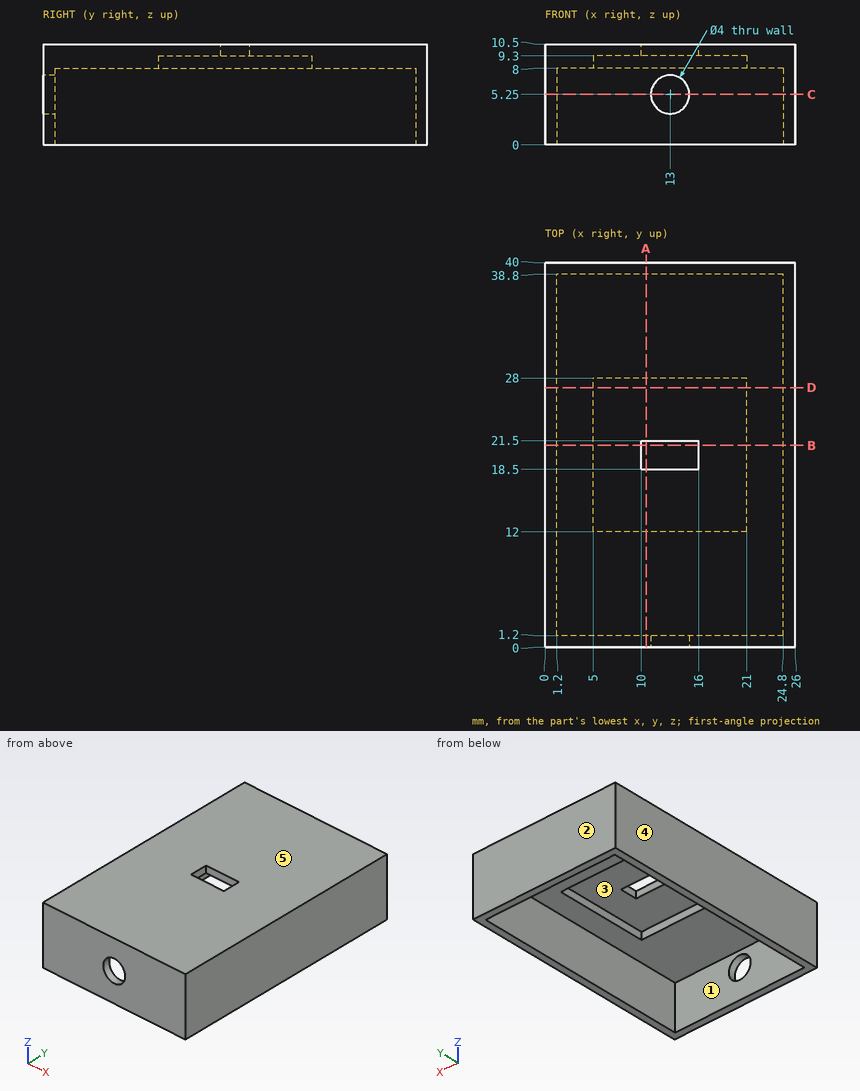
Study the drawing (mm; zero at the part's minimum x, y, z) and answer. A direction names the side the tool comes from. Round coordinates to 2 decimals unless told otherwise and drop trailing zeros. Order: outer loops, then holes, each group sorted by start corner. A loop starts at its lowest first (then second) coordinate and runs counter-clockwise, first axis right, second up. Notation, with made-up numbers: M -2,50.25 L 2,50.25 A32 cw 2,86.25 Z; hole C -7,59 d6. An arc over 180 degrees is marked long. One line per item, written item: value.
Q1. Flat-ended cylindrical pins translate along their axes: pin 1 (5 mm diameter, centred on x = 20, y = 17, fed in from -Z); pin 2 (5 mm diameter, centred on x = 16, y = 23.5, fed in from -Z). Find the tip coordinate at first contact, or state that the pin passes through.
Derived:
pin 1: z = 8
pin 2: z = 9.3
Q2. Determine the mould class of the marked faces 3, 4 and 5 for opening direction X: released by +X, released by -X, zero draft, split by the parting line, or undercut.
Derived:
face 3: undercut
face 4: released by -X
face 5: zero draft
Q3. Find section B-B on y = 21. Write down the section's boundary in (x, z), then the cut area to 3 significant figures.
Derived:
outline: M 0,0 L 1.2,0 L 1.2,8 L 5,8 L 5,9.3 L 10,9.3 L 10,10.5 L 0,10.5 Z; M 16,9.3 L 21,9.3 L 21,8 L 24.8,8 L 24.8,0 L 26,0 L 26,10.5 L 16,10.5 Z
area: 56.2 mm²
Q4. For the marked faces 1 and 2, determine the directions among +Z, -Z, +X, -X, +Y, -Y from which every point of the face is accessible in a straight line to the end or side of a thin tool.
Derived:
face 1: -Z
face 2: +Z, -Z, +X, -X, +Y
Q5. Find section D-D on y = 27. Write down the section's boundary in (x, z), then the cut area to 3 significant figures.
Derived:
outline: M 0,0 L 1.2,0 L 1.2,8 L 5,8 L 5,9.3 L 21,9.3 L 21,8 L 24.8,8 L 24.8,0 L 26,0 L 26,10.5 L 0,10.5 Z
area: 63.4 mm²
Q6. Find section C-C on z = 5.25. Write down the section's boundary in (x, y), then the cut area to 3 significant figures.
Derived:
outline: M 0,0 L 11,0 L 11,1.2 L 1.2,1.2 L 1.2,38.8 L 24.8,38.8 L 24.8,1.2 L 15,1.2 L 15,0 L 26,0 L 26,40 L 0,40 Z
area: 148 mm²
Q7. Straight lines are drawn through the part: line 1 (X direction, y = 0.65, z = 5.25); line 2 (Y direction, x = 7, z = 6.5); line 3 (X direction, y = 11.5, z = 1.25). For each, find the intervals that lie inside material, in ascending order.
Derived:
line 1: 0 to 11, 15 to 26
line 2: 0 to 1.2, 38.8 to 40
line 3: 0 to 1.2, 24.8 to 26
Q8. Find section A-A on x = 10.5. Write down the section's boundary in (y, z).
Derived:
outline: M 0,0 L 1.2,0 L 1.2,8 L 12,8 L 12,9.3 L 18.5,9.3 L 18.5,10.5 L 0,10.5 Z; M 21.5,9.3 L 28,9.3 L 28,8 L 38.8,8 L 38.8,0 L 40,0 L 40,10.5 L 21.5,10.5 Z
